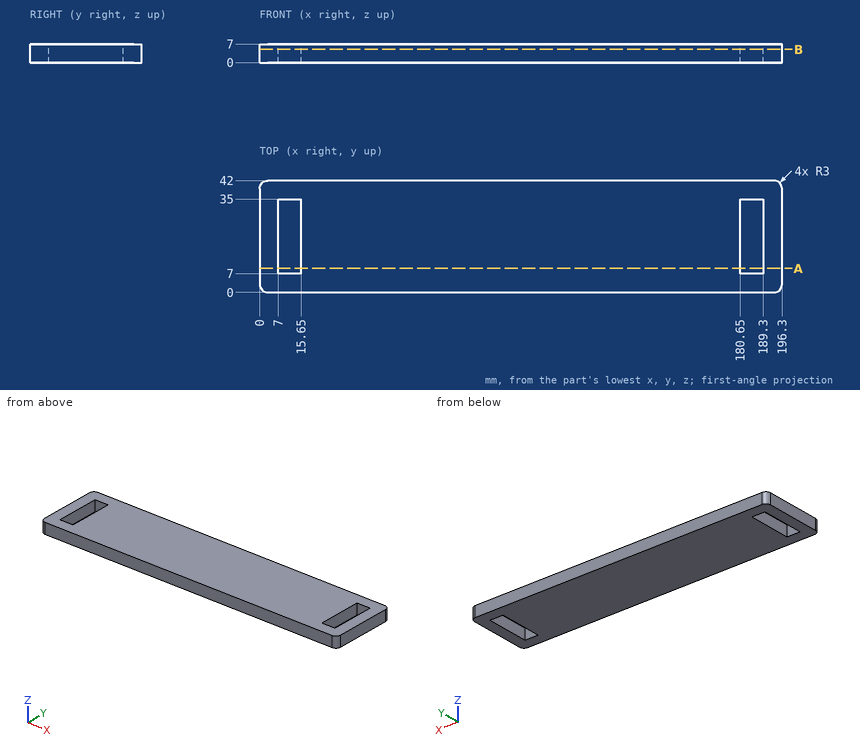
Design review of the part shown in the three views and the two pictorial views. Dimensions are in mm from the part's minimum x, y and z. Give positions to 0.01 mm unless a question says otherwise; leave off trailing zeros. Write each loop counter-clockwise with the first axis right and the second up, starting at its lowest first coordinate (ties: lowest second). Pieces come first, ordered by that corner, then holes. Notation, with made-up numbers: M 62,16 L 68,16 A20 cw 68,50 Z; hole C -16,69 d6. An arc over 180 degrees is marked long. Answer in a Markdown table with one row per item.
Item 1: Add section B-B on z = 5. Give the boundary of the cut face in (x, y), plus the area to 3 significant figures.
Check sheet entries:
| item | result |
|---|---|
| outline | M 0,3 A3 ccw 3,0 L 193.3,0 A3 ccw 196.3,3 L 196.3,39 A3 ccw 193.3,42 L 3,42 A3 ccw 0,39 Z; hole M 7,7 L 15.65,7 L 15.65,35 L 7,35 Z; hole M 180.65,7 L 189.3,7 L 189.3,35 L 180.65,35 Z |
| area | 7,750 mm2 |
Item 2: Add section A-A on y = 9. Give the boundary of the cut face in (x, z).
Check sheet entries:
| item | result |
|---|---|
| outline | M 0,0 L 7,0 L 7,7 L 0,7 Z; M 15.65,0 L 180.65,0 L 180.65,7 L 15.65,7 Z; M 189.3,0 L 196.3,0 L 196.3,7 L 189.3,7 Z |
Item 3: For line 1 along X through (y, z) = (13, 2.25); line 2 along Y through (x, z) = (182.5, 6.75), list the stretches that pass through material, from the lowest coordinate up.
Check sheet entries:
| item | result |
|---|---|
| line 1 | 0 to 7, 15.65 to 180.65, 189.3 to 196.3 |
| line 2 | 0 to 7, 35 to 42 |
